Answer from the drawing. Dimensions are ordinates in mm from the lowest x, y and z of the part. A direction names the side the tool comes from. Coordinates: 2 decimals unless noted, no trailing zeros. Loops run counter-clockwise (first coordinate to the right, second up) from the corner with the lowest first, then second, coordinate; pieces in that order, holes last. Notation, with made-up numbers: (-14.5, -11.5) -> (12.5, -11.5) arc R12 ccw to (12.5, -3.5) -> close; hole circle Ø2 at (39, 89). An arc over 180 degrees is marked (long way). Use a Markdown table: item, result.
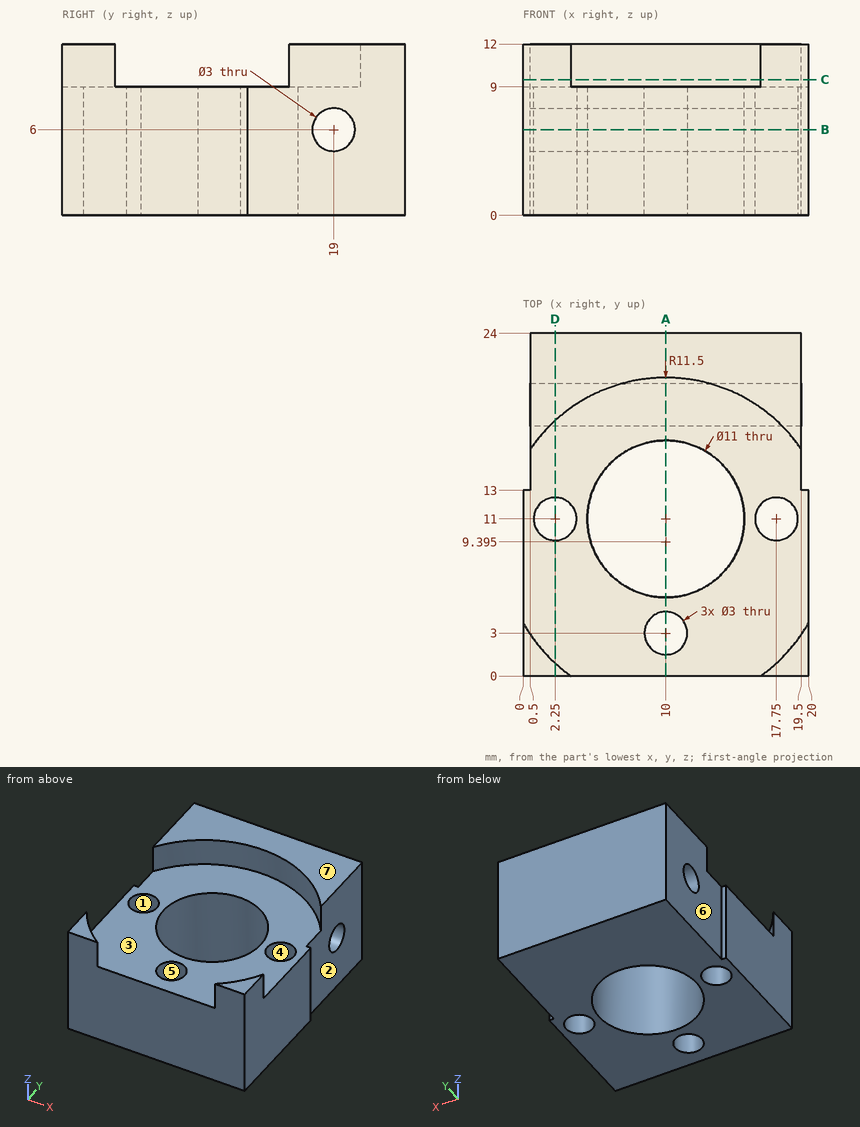
Q1. For the marked faces 1, 2 and 3, determine the directions among +Z, -Z, +X, -X, +Y, -Y from which every point of the face is accessible in a straight line to the end or side of a thin tool.
Solved:
| item | result |
|---|---|
| face 1 | +Z, -Z |
| face 2 | +Z, -Z, +X, +Y |
| face 3 | +Z |
Q2. Consider line 1 (Y direction, x = 10, z = 2); line 2 (Y direction, x = 10, z = 6.25); line 3 (Y direction, x = 10, z = 6.5). Determine where each line is inside the solid, lowest interval first. Write a range as [from, to].
Solved:
| item | result |
|---|---|
| line 1 | [0, 1.5], [4.5, 5.5], [16.5, 24] |
| line 2 | [0, 1.5], [4.5, 5.5], [16.5, 17.52], [20.48, 24] |
| line 3 | [0, 1.5], [4.5, 5.5], [16.5, 17.59], [20.41, 24] |
Q3. Section B-B on z = 6 is taken. Determine the outline of the cut face in (x, y).
Solved:
| item | result |
|---|---|
| outline | (0, 0) -> (20, 0) -> (20, 13) -> (19.5, 13) -> (19.5, 17.5) -> (0.5, 17.5) -> (0.5, 13) -> (0, 13) -> close; (0.5, 20.5) -> (19.5, 20.5) -> (19.5, 24) -> (0.5, 24) -> close; hole circle Ø3 at (2.25, 11); hole circle Ø11 at (10, 11); hole circle Ø3 at (10, 3); hole circle Ø3 at (17.75, 11) |
Q4. Given pin 1 Ø10 at (x, y) = (10.5, 13.5) entering from +Z; pin 2 Ø2.5 at (x, y) = (10, 3) entering from +Z; pin 3 Ø5.5 at (y, z) = (16, 6) entering from -X, each flat-ended and moving along its own axis, determine where each tip first touches the part or whether it passes through.
Solved:
| item | result |
|---|---|
| pin 1 | z = 9 |
| pin 2 | through |
| pin 3 | x = 0.5 |
Q5. Section D-D on x = 2.25 is taken. Determine the outline of the cut face in (y, z), and give its area (3 significant figures).
Solved:
| item | result |
|---|---|
| outline | (0, 0) -> (9.5, 0) -> (9.5, 9) -> (0.9, 9) -> (0.9, 12) -> (0, 12) -> close; (12.5, 0) -> (24, 0) -> (24, 12) -> (17.89, 12) -> (17.89, 9) -> (12.5, 9) -> close; hole circle Ø3 at (19, 6) |
| area | 203 mm² |
Q6. Section A-A on x = 10 is taken. Determine the outline of the cut face in (y, z) (1 decimal).
Solved:
| item | result |
|---|---|
| outline | (0, 0) -> (1.5, 0) -> (1.5, 9) -> (0, 9) -> close; (4.5, 0) -> (5.5, 0) -> (5.5, 9) -> (4.5, 9) -> close; (16.5, 0) -> (24, 0) -> (24, 12) -> (20.9, 12) -> (20.9, 9) -> (16.5, 9) -> close; hole circle Ø3 at (19, 6) |
Q7. Section C-C on z = 9.5 is taken. Determine the outline of the cut face in (x, y) (1 decimal).
Solved:
| item | result |
|---|---|
| outline | (0, 0) -> (3.4, 0) arc R11.5 cw to (0, 3.7) -> close; (0.5, 15.9) arc R11.5 cw to (19.5, 15.9) -> (19.5, 24) -> (0.5, 24) -> close; (16.6, 0) -> (20, 0) -> (20, 3.7) arc R11.5 cw to start |
Q8. Determine the mould class of the marked faces 4, 5, 6 and 7 for opening direction X: pulls with the +X half, pulls with the -X half, needs draft (parallel to the pull), parting line crosses it, or undercut.
Solved:
| item | result |
|---|---|
| face 4 | undercut |
| face 5 | undercut |
| face 6 | pulls with the -X half |
| face 7 | needs draft |
